Autodesk Inventor part; units mm, degrees
ref_plane "YZ Plane" through (0, 0, 0) normal (1, 0, 0) x (0, 1, 0)
ref_plane "XZ Plane" through (0, 0, 0) normal (0, 1, 0) x (-1, 0, 0)
ref_plane "XY Plane" through (0, 0, 0) normal (0, 0, 1) x (1, 0, 0)
sketch "Sketch1" plane through (0, 0, 0) normal (1, 0, 0) x (0, 1, 0)
  line L0 (0, 0) -> (0, -120)
  line L1 (0, -120) -> (50, -96.6846)
  line L2 (0, 0) -> (50, -23.3154)
  line L3 (50, -23.3154) -> (50, -96.6846)
  dimension "d0" = 120
  dimension "d1" = 65
  dimension "d2" = 65
  dimension "d3" = 50
  dimension "d4" = 50
extrude "Extrusion1" add sketch "Sketch1" along normal blind 70
shell "Shell1" thickness 3 removed faces 2 at (23.3333, 50, -72.2282) at (23.3333, 0, -40)
sketch "Sketch2" plane through (0, 50, -23.3154) normal (0, 1, 0) x (1, 0, 0)
  line L0 (35, 37.1714) -> (45, 37.1714) construction
  line L1 (35, 37.1714) -> (25, 37.1714) construction
  line L2 (0, 96.6846) -> (70, 96.6846)
  line L3 (25, 96.6846) -> (25, -23.3154)
  line L4 (0, -23.3154) -> (70, -23.3154)
  line L5 (45, 96.6846) -> (45, -23.3154)
  line L6 (45, -23.3154) -> (25, -23.3154)
  line L7 (25, 96.6846) -> (45, 96.6846)
  point P0 (45, -23.3154)
  dimension "d8" = 10
  dimension "d9" = 10
  dimension "d10" = 20
extrude "Extrusion2" cut sketch "Sketch2" against normal blind 40
properties part number "Pie_3DPrint"
Input: part model. Units: mm. Frame: model coordinates. A direction names the side the tool comes from. Round coordinates to 2 decimals unless told otherwise and drop trailing zeros. Write each loop counter-clockwise with the first axis right and the second up, starting at its lowest first coordinate (ties: lowest second). Pieces come first, ordered by that corner, then holes. Notation, with made-up numbers: M 51,37 L 61,37 A11 ccw 61,43 Z; hole C 2.25,-3.5 d7. An arc over 180 degrees is marked long. Write each question's results on one line, items separated by ' | '.
Q1. Draft query along Z for faces 1 (the face through (18.954, 24.65, -11.494)), 2 (the face through (69, 0, -55)), 3 (the face through (48.774, 24.65, -105.195)). Return one class per face: released by +Z, released by -Z, zero draft, split by the parting line, or undercut.
Results:
face 1: released by +Z | face 2: zero draft | face 3: undercut
Q2. Section query B-B (x = 43). Return loops of the section in (y, z).
Results:
outline: M 0,-120 L 10,-115.34 L 10,-112.03 L 0,-116.69 Z; M 0,-3.31 L 10,-7.97 L 10,-4.66 L 0,0 Z
Q3. Section query D-D (y = 4.5). Return loops of the section in (x, z).
Results:
outline: M 0,-117.9 L 70,-117.9 L 70,-2.1 L 0,-2.1 Z; hole M 3,-114.59 L 67,-114.59 L 67,-5.41 L 3,-5.41 Z
Q4. Section query C-C (y = 37). Return loops of the section in (x, z), and give its area (3 significant figures).
Results:
outline: M 0,-102.75 L 25,-102.75 L 25,-99.44 L 3,-99.44 L 3,-20.56 L 25,-20.56 L 25,-17.25 L 0,-17.25 Z; M 45,-102.75 L 70,-102.75 L 70,-17.25 L 45,-17.25 L 45,-20.56 L 67,-20.56 L 67,-99.44 L 45,-99.44 Z | area: 804 mm^2
Q5. Line query: line 1 along X through (y, z) = (28, -19.5); line 2 along Z through (x, y) = (22, 8.5); line 3 along Z through (x, y) = (49, 18). Output: solid intervals per line, ascending.
Results:
line 1: x = 0 to 3, 67 to 70 | line 2: z = -116.04 to -112.73, -7.27 to -3.96 | line 3: z = -111.61 to -108.3, -11.7 to -8.39
Q6. Pin query (flat end, axial travel): P1, Ø1.7, axis at x = 33.5, z = -113.5, coming from the +Y side; P2, Ø1.5, axis at x = 48, y = 37, coming from the +Z side; P3, Ø5, axis at x = 18, y = 14, coming from the +Z side; P4, Ø11, axis at y = 22, z = -102.5, coming from the -X side. Return the tip coordinate at first contact, or that it passes through.
Results:
P1: stops at y = 10 | P2: stops at z = -16.9 | P3: stops at z = -5.36 | P4: stops at x = 0
Q7. Section query A-A (z = -78.5). Return loops of the section in (x, y).
Results:
outline: M 0,0 L 3,0 L 3,50 L 0,50 Z; M 67,0 L 70,0 L 70,50 L 67,50 Z
Q8. Access query for faces 4 (the face through (35, 10, -6)), 5 (the face through (70, 25, -59)), 6 (the face through (67, 25, -59)). Directions: +Z, -Z, +X, -X, +Y, -Y. A direction counts if a zero-diameter tool reaches every point of the face in a straight line with its end or side. Return the directions, or none.
Results:
face 4: +Z, -Z, +Y | face 5: +Z, -Z, +X, +Y, -Y | face 6: -Y
